from build123d import *

# Parameters (mm, degrees)
SKETCH_1_W               = 70
SKETCH_1_H               = 35
EXTRUDE_1_DEPTH          = 25
SKETCH_3_R               = 12.5
CUT_EXTRUDE_2_DEPTH      = 20
SKETCH_5_R               = 6.75
CUT_EXTRUDE_4_DEPTH      = 5
SKETCH_6_R               = 1.6
CUT_EXTRUDE_5_DEPTH      = 5
SKETCH_8_R               = 12.5
CUT_EXTRUDE_6_DEPTH      = 20
SKETCH_9_R               = 6.75
CUT_EXTRUDE_7_DEPTH      = 20
SKETCH_10_R              = 1.6
CUT_EXTRUDE_8_DEPTH      = 44.945989578
SKETCH_11_R              = 3.4
CUT_EXTRUDE_9_DEPTH      = 56.452682532
EXTRUDE_START            = 3
SKETCH_13_W              = 70
SKETCH_13_H              = 25
SKETCH_13_R              = 3.4
EXTRUDE_3_DEPTH          = 3
SKETCH_2_R               = 2.1
CUT_EXTRUDE_1_DEPTH      = 58.393379519
SKETCH_15_W              = 25
SKETCH_15_H              = 38
EXTRUDE_4_DEPTH          = 5
SKETCH_16_W              = 25
SKETCH_16_H              = 38
EXTRUDE_5_DEPTH          = 5
SKETCH_17_R              = 2.1
CUT_EXTRUDE_11_DEPTH     = 61.572270988
SKETCH_18_R              = 1.25
CUT_EXTRUDE_12_DEPTH     = 5
MIRROR_2_COPY_1_SKETCH_R = 1.25
MIRROR_2_COPY_1_DEPTH    = 5


with BuildPart() as part:
    # 草图1 → 凸台-拉伸1 (new body)
    with BuildSketch(Plane.XY):
        Rectangle(SKETCH_1_W, SKETCH_1_H)
    extrude(amount=EXTRUDE_1_DEPTH)

    # 草图3 → 切除-拉伸2 (cut)
    with BuildSketch(Plane(origin=(0, 0, 0), x_dir=(-1, 0, 0), z_dir=(0, 0, -1))):
        with Locations((15, 0)):
            Circle(SKETCH_3_R)
    extrude(amount=-CUT_EXTRUDE_2_DEPTH, mode=Mode.SUBTRACT)

    # 草图5 → 切除-拉伸4 (cut)
    with BuildSketch(Plane(origin=(0, 0, 20), x_dir=(-1, 0, 0), z_dir=(0, 0, -1))):
        with Locations((15, 0)):
            Circle(SKETCH_5_R)
    extrude(amount=-CUT_EXTRUDE_4_DEPTH, mode=Mode.SUBTRACT)

    # 草图6 → 切除-拉伸5 (cut)
    with BuildSketch(Plane(origin=(0, 0, 20), x_dir=(-1, 0, 0), z_dir=(0, 0, -1))):
        with Locations((15, -9.5)):
            Circle(SKETCH_6_R)
        with Locations((6.772758664, 4.75)):
            Circle(SKETCH_6_R)
        with Locations((23.227241336, 4.75)):
            Circle(SKETCH_6_R)
    extrude(amount=-CUT_EXTRUDE_5_DEPTH, mode=Mode.SUBTRACT)

    # 草图8 → 切除-拉伸6 (cut)
    with BuildSketch(Plane.XY.offset(25)):
        with Locations((15, 0)):
            Circle(SKETCH_8_R)
    extrude(amount=-CUT_EXTRUDE_6_DEPTH, mode=Mode.SUBTRACT)

    # 草图9 → 切除-拉伸7 (cut)
    with BuildSketch(Plane.XY.offset(5)):
        with Locations((15, 0)):
            Circle(SKETCH_9_R)
    extrude(amount=-CUT_EXTRUDE_7_DEPTH, mode=Mode.SUBTRACT)

    # 草图10 → 切除-拉伸8 (cut, through all)
    with BuildSketch(Plane.XY.offset(5)):
        with Locations((15, -9.5)):
            Circle(SKETCH_10_R)
        with Locations((6.772758664, 4.75)):
            Circle(SKETCH_10_R)
        with Locations((23.227241336, 4.75)):
            Circle(SKETCH_10_R)
    extrude(amount=-CUT_EXTRUDE_8_DEPTH, mode=Mode.SUBTRACT)

    # 草图11 → 切除-拉伸9 (cut, through all)
    with BuildSketch(Plane.XZ.offset(17.5)):
        with Locations(Location((22, 12.5, 0), (0, 0, 270))):
            Circle(SKETCH_11_R)
        with Locations(Location((-22, 12.5, 0), (0, 0, 270))):
            Circle(SKETCH_11_R)
    extrude(amount=-CUT_EXTRUDE_9_DEPTH, mode=Mode.SUBTRACT)

    # 草图13 → 凸台-拉伸3 (add)
    with BuildSketch(Plane.XZ.offset(17.5).offset(EXTRUDE_START)):
        with Locations((0, 12.5)):
            Rectangle(SKETCH_13_W, SKETCH_13_H)
        with Locations(Location((-22, 12.5, 0), (0, 0, 270))):
            Circle(SKETCH_13_R, mode=Mode.SUBTRACT)
        with Locations(Location((22, 12.5, 0), (0, 0, 270))):
            Circle(SKETCH_13_R, mode=Mode.SUBTRACT)
    extrude(amount=-EXTRUDE_3_DEPTH)

    # 草图2 → 切除-拉伸1 (cut, through all)
    with BuildSketch(Plane(origin=(0, 17.5, 0), x_dir=(1, 0, 0), z_dir=(0, 1, 0))):
        with Locations(Location((30, -5, 0), (0, 0, 270))):
            Circle(SKETCH_2_R)
        with Locations(Location((30, -20, 0), (0, 0, 270))):
            Circle(SKETCH_2_R)
        with Locations(Location((-30, -5, 0), (0, 0, 270))):
            Circle(SKETCH_2_R)
        with Locations(Location((-30, -20, 0), (0, 0, 270))):
            Circle(SKETCH_2_R)
    extrude(amount=-CUT_EXTRUDE_1_DEPTH, mode=Mode.SUBTRACT)

    # 草图15 → 凸台-拉伸4 (add)
    with BuildSketch(Plane.ZY.offset(35)):
        with Locations((12.5, -1.5)):
            Rectangle(SKETCH_15_W, SKETCH_15_H)
    extrude(amount=EXTRUDE_4_DEPTH)

    # 草图16 → 凸台-拉伸5 (add)
    with BuildSketch(Plane(origin=(35, 0, 0), x_dir=(0, 0, -1), z_dir=(1, 0, 0))):
        with Locations((-12.5, -1.5)):
            Rectangle(SKETCH_16_W, SKETCH_16_H)
    extrude(amount=EXTRUDE_5_DEPTH)

    # 草图17 → 切除-拉伸11 (cut, through all)
    with BuildSketch(Plane.XZ.offset(20.5)):
        with Locations(Location((0, 5, 0), (0, 0, 270))):
            Circle(SKETCH_17_R)
        with Locations(Location((0, 20, 0), (0, 0, 90))):
            Circle(SKETCH_17_R)
    extrude(amount=-CUT_EXTRUDE_11_DEPTH, mode=Mode.SUBTRACT)

    # 草图18 → 切除-拉伸12 (cut)
    with BuildSketch(Plane(origin=(0, 0, 0), x_dir=(-1, 0, 0), z_dir=(0, 0, -1))):
        with Locations((-37, 7.5)):
            Circle(SKETCH_18_R)
        with Locations((-37, -2.5)):
            Circle(SKETCH_18_R)
    cut_extrude_12 = extrude(amount=-CUT_EXTRUDE_12_DEPTH, mode=Mode.SUBTRACT)

    # 镜向1: 切除-拉伸12 across plane
    add(cut_extrude_12.mirror(Plane.XY.offset(12.5)), mode=Mode.SUBTRACT)

    # 镜向2: 切除-拉伸12 across plane
    add(cut_extrude_12.mirror(Plane(origin=(0, 0, 0), x_dir=(0, 0, 1), z_dir=(1, 0, 0))), mode=Mode.SUBTRACT)

    # 镜向2 copy 1 sketch → 镜向2 copy 1 (cut)
    with BuildSketch(Plane.XY.offset(25)):
        with Locations((-37, 7.5)):
            Circle(MIRROR_2_COPY_1_SKETCH_R)
        with Locations((-37, -2.5)):
            Circle(MIRROR_2_COPY_1_SKETCH_R)
    extrude(amount=-MIRROR_2_COPY_1_DEPTH, mode=Mode.SUBTRACT)


solid = part.part
The listing builds one solid part. Answer for the finished solid, in the listing's coordinates (mm). A direction names the side the tool comes from. Give positions to 0.01 mm unless a question says otherwise; leave off trailing zeros. Loops run counter-clockwise (first coordinate to the right, second up) from the corner with the lowest first, then second, coordinate; pieces in that order, holes last. Notation, with made-up numbers: (87, 78.25) - (125, 78.25) arc R20 ccw to (125, 115.25) - close; hole circle Ø8 at (-16.75, 70). An arc over 180 degrees is marked (long way). Answer as a JSON object with one key per item and string values.
1. A cutting plane is placed at A-A (y = -6). Give the number of separate pieces and of enclosed holes in the cut face, then the cut area to 3 significant figures.
Determined:
{"separate pieces": "3", "enclosed holes": "6", "area": "978 mm²"}
2. A cutting plane is placed at D-D (z = 12.5). Write down the section's boundary in (x, y).
Determined:
{"outline": "(-40, -20.5) - (-25.4, -20.5) - (-25.4, -6.93) arc R12.5 cw to (-25.4, 6.93) - (-25.4, 17.5) - (-40, 17.5) - close; (-18.6, -20.5) - (18.6, -20.5) - (18.6, -11.97) arc R12.5 cw (long way) to (18.6, 11.97) - (18.6, 17.5) - (-18.6, 17.5) - (-18.6, 11.97) arc R12.5 cw (long way) to (-18.6, -11.97) - close; (25.4, -20.5) - (40, -20.5) - (40, 17.5) - (25.4, 17.5) - (25.4, 6.93) arc R12.5 cw to (25.4, -6.93) - close"}
3. A cutting plane is placed at B-B (x = 0). Write down the section's boundary in (y, z), then the cut area to 3 significant figures.
Determined:
{"outline": "(-20.5, 0) - (17.5, 0) - (17.5, 2.9) - (-20.5, 2.9) - close; (-20.5, 7.1) - (17.5, 7.1) - (17.5, 17.9) - (-20.5, 17.9) - close; (-20.5, 22.1) - (17.5, 22.1) - (17.5, 25) - (-20.5, 25) - close", "area": "631 mm²"}
4. Find the intervals of material crossed by L1, parallel to Y at x = -37, z = 1.3; L2, parallel to Y at x = -15, z = 21.5; L3, parallel to Z at x = 22, y = -13, in increasing order. Write a range as [from, to].
Determined:
{"L1": "[-20.5, -3.75], [-1.25, 6.25], [8.75, 17.5]", "L2": "[-20.5, -11.1], [-7.9, -6.75], [6.75, 17.5]", "L3": "[0, 9.1], [15.9, 25]"}
5. For a pull along X with two mould halves and no side action, classify faces 4 (the flat face through (-40, -1, 12)), 5 (the cylindrical face through (-13.73, -10.47, 22.46)) as pulls with the +X half, pulls with the -X half, needs draft (parallel to the pull), parting line crosses it, or undercut.
Determined:
{"face 4": "pulls with the -X half", "face 5": "undercut"}
6. Flat-ended cylindrical pins translate along their axes: pin 1 Ø5 at (x, z) = (30, 20) entering from +Y; pin 2 Ø12.5 at (x, y) = (-16.5, -3.5) entering from -Z; pin 3 Ø2 at (x, y) = (-37, -2.5) entering from +Z; pin 4 Ø2 at (x, y) = (-37, 7.5) entering from -Z. Find the tip coordinate at first contact, or state that the pin passes through.
Determined:
{"pin 1": "y = 17.5", "pin 2": "z = 20", "pin 3": "z = 20", "pin 4": "z = 5"}
7. For faces 1 (the cylindrical face through (21.438, 2.028, 2.535)), 2 (the cylindrical face through (-38.25, -2.45, 22.54)), 3 (the cylindrical face through (-37.99, 6.74, 2.46)), determine the directions among +Z, -Z, +X, -X, +Y, -Y from which every point of the face is accessible in a straight line to the end or side of a thin tool.
Determined:
{"face 1": "+Z, -Z", "face 2": "+Z", "face 3": "-Z"}
